Geometry: final body of the model. Coordinates: model frame, mm. A direction names the side the tool comes from. Give positions to 0.01 mm unless a question says otherwise; leave off trailing zeros. Order: outer loops, then holes, each group sorted by start corner. A loop starts at its lowest first (then second) coordinate and runs counter-clockwise, first axis right, second up. Notation, with made-up numbers: (-39.5, 75.5) - (-3.5, 75.5) arc R19 cw to (-3.5, 106.5) - close; hole circle Ø1 at (22, 49). An arc over 180 degrees is marked (long way). Use one line per item in the form item = value.
from build123d import *

# Parameters (mm, degrees)
F1_DEPTH = 20
F2_W     = 10
F2_H     = 40
F3_DEPTH = 30
F4_W     = 2
F4_H     = 18
F4_H_2   = 2
F4_W_2   = 18
F5_DEPTH = 30


# Not quite as in the source:
# - a feature names something its author has since deleted; it is built from what else it names


with BuildPart() as f1:
    # F0 (on Front) → F1 (new body, symmetric)
    with BuildSketch(Plane.XZ):
        with BuildLine():
            Line((-10, -5), (20, -5))
            Line((20, -5), (20, 5))
            Line((20, 5), (-20, 5))
            ThreePointArc((-20, 5), (-27.0710678119, 2.0710678119), (-30, -5))
            Line((-30, -5), (-30, -37.0084848255))
            Line((-30, -37.0084848255), (-29.9999700785, -37.1900333921))
            ThreePointArc((-29.9999700785, -37.1900333921), (-27.134358967, -44.1955599538), (-20.1815186475, -47.1867371371))
            Line((-20.1815186475, -47.1867371371), (-20, -47.1900331229))
            Line((-20, -47.1900331229), (-10, -47.1900331229))
            Line((-10, -47.1900331229), (-6.8265195005, -47.1900331229))
            ThreePointArc((-6.8265195005, -47.1900331229), (0.2445483114, -44.2611009348), (3.1734804995, -37.1900331229))
            Line((3.1734804995, -37.1900331229), (3.1734804995, -32.0262350142))
            Line((3.1734804995, -32.0262350142), (20, -32.0262350142))
            Line((20, -32.0262350142), (20, -27.0262350142))
            ThreePointArc((20, -27.0262350142), (18.5355339059, -23.4907011083), (15, -22.0262350142))
            Line((15, -22.0262350142), (3.1734804995, -22.0262350142))
            Line((3.1734804995, -22.0262350142), (-1.7689520504, -22.0262350142))
            ThreePointArc((-1.7689520504, -22.0262350142), (-5.3044859563, -23.4907011083), (-6.7689520504, -27.0262350142))
            Line((-6.7689520504, -27.0262350142), (-6.7689520504, -32.0262350142))
            ThreePointArc((-6.7689520504, -32.0262350142), (-8.2395588674, -35.5501802143), (-11.7686128262, -37.0084848255))
            Line((-11.7686128262, -37.0084848255), (-15, -37.0084848255))
            ThreePointArc((-15, -37.0084848255), (-18.5355339059, -35.5440187314), (-20, -32.0084848255))
            Line((-20, -32.0084848255), (-20, -15))
            Line((-20, -15), (-20, -10))
            ThreePointArc((-20, -10), (-18.5355339059, -6.4644660941), (-15, -5))
            Line((-15, -5), (-10, -5))
        make_face()
    extrude(amount=F1_DEPTH, both=True)

    # F2 (on face) → F3 (join)
    with BuildSketch(Plane.XY.offset(5)):
        with Locations((5, 0)):
            Rectangle(F2_W, F2_H)
        with Locations((-5, 0)):
            Rectangle(F2_W, F2_H)
        with Locations((-15, 0)):
            Rectangle(F2_W, F2_H)
        with Locations((15, 0)):
            Rectangle(F2_W, F2_H)
    extrude(amount=F3_DEPTH)

    # F4 (on face) → F5 (cut)
    with BuildSketch(Plane.XY.offset(35)):
        with Locations((-1, 11)):
            Rectangle(F4_W, F4_H)
        with Locations((-1, 1)):
            Rectangle(F4_W, F4_H_2)
        with Locations((-1, -1)):
            Rectangle(F4_W, F4_H_2)
        with Locations((-1, -11)):
            Rectangle(F4_W, F4_H)
        with Locations((1, 11)):
            Rectangle(F4_W, F4_H)
        with Locations((1, 1)):
            Rectangle(F4_W, F4_H_2)
        with Locations((1, -1)):
            Rectangle(F4_W, F4_H_2)
        with Locations((1, -11)):
            Rectangle(F4_W, F4_H)
        with Locations((11, 1)):
            Rectangle(F4_W_2, F4_H_2)
        with Locations((11, -1)):
            Rectangle(F4_W_2, F4_H_2)
        with Locations((-11, -1)):
            Rectangle(F4_W_2, F4_H_2)
        with Locations((-11, 1)):
            Rectangle(F4_W_2, F4_H_2)
    extrude(amount=-F5_DEPTH, mode=Mode.SUBTRACT)


solid = f1.part
(1) Cut plane C-C on z = -12.5. Output: boundary loops of the cut face in (x, y), plus the area to 3 significant figures.
Computed values:
outline = (-30, -20) - (-20, -20) - (-20, 20) - (-30, 20) - close
area = 400 mm²
(2) Cut plane D-D on y = 1. Output: boundary loops of the cut face in (x, z).
Computed values:
outline = (-30, -37.19) arc R10 ccw to (-20.18, -47.19) - (-20, -47.19) - (-6.83, -47.19) arc R10 ccw to (3.17, -37.19) - (3.17, -32.03) - (20, -32.03) - (20, -27.03) arc R5 ccw to (15, -22.03) - (-1.77, -22.03) arc R5 ccw to (-6.77, -27.03) - (-6.77, -32.03) arc R5 cw to (-11.77, -37.01) - (-15, -37.01) arc R5 cw to (-20, -32.01) - (-20, -10) arc R5 cw to (-15, -5) - (20, -5) - (20, 5) - (-20, 5) arc R10 ccw to (-30, -5) - (-30, -37.01) - close
(3) Pull-direction query (X, two-part tool) for faces 1 (the face through (-2, -11, 20)), 2 (the face through (2, 0, -5)), 3 (the face through (-20, -11, 20)), 4 (the face through (3.173, 0, -35)); classes: released by +X, released by -X, zero draft, split by the parting line, or undercut.
Computed values:
face_1 = undercut
face_2 = zero draft
face_3 = released by -X
face_4 = released by +X
(4) Reachability of faces 5 (the face through (-11, 11, 35)), 6 (the face through (-14, 0, -47.19)), 7 (the face through (-13, 0, -37.008)), 8 (the face through (-11, -2, 20)), 9 (the face through (18.574, -0.28, -23.53)) from +Z, -Z, +X, -X, +Y, -Y: full face, straight path, thin tool, end or side. Return the list, or none.
Computed values:
face_5 = +Z, +X, -X, +Y, -Y
face_6 = -Z, +X, -X, +Y, -Y
face_7 = +Y, -Y
face_8 = +Z, +X, -X
face_9 = +X, +Y, -Y
(5) Cut plane B-B on y = 11. Output: boundary loops of the cut face in (x, z).
Computed values:
outline = (-30, -37.19) arc R10 ccw to (-20.18, -47.19) - (-20, -47.19) - (-6.83, -47.19) arc R10 ccw to (3.17, -37.19) - (3.17, -32.03) - (20, -32.03) - (20, -27.03) arc R5 ccw to (15, -22.03) - (-1.77, -22.03) arc R5 ccw to (-6.77, -27.03) - (-6.77, -32.03) arc R5 cw to (-11.77, -37.01) - (-15, -37.01) arc R5 cw to (-20, -32.01) - (-20, -10) arc R5 cw to (-15, -5) - (20, -5) - (20, 35) - (2, 35) - (2, 5) - (-2, 5) - (-2, 35) - (-20, 35) - (-20, 5) arc R10 ccw to (-30, -5) - (-30, -37.01) - close
(6) Cut plane A-A on x = 10. Output: boundary loops of the cut face in (y, z), plus the area to 3 significant figures.
Computed values:
outline = (-20, -32.03) - (20, -32.03) - (20, -22.03) - (-20, -22.03) - close; (-20, -5) - (20, -5) - (20, 35) - (2, 35) - (2, 5) - (-2, 5) - (-2, 35) - (-20, 35) - close
area = 1,880 mm²
(7) Contact query for flat-ended pins moving along their axis: pin 1 Ø9 at (y, z) = (-8.5, 23.5) entering from -X; pin 2 Ø2.5 at (x, y) = (-14, -0.5) entering from +Z; pin 3 Ø18.5 at (x, y) = (11, 5.5) entering from -Z; pin 4 Ø8 at (x, z) = (-25, 12.5) entering from +Y. Output: stop coordinate, or through.
Computed values:
pin_1 = -20
pin_2 = 5
pin_3 = -42.33
pin_4 = through
(8) Ray query, line 1 along Y through (x, z) = (10, 17.5); line 2 along Z through (x, y) = (13.5, -17.5). Return the intervals inside material, ascending.
Computed values:
line_1 = -20 to -2, 2 to 20
line_2 = -32.03 to -22.03, -5 to 35
